```python
from build123d import *

# Parameters (mm, degrees)
BOSS_EXTRUDE1_DEPTH = 12.5
BOSS_EXTRUDE2_DEPTH = 7.5
BOSS_EXTRUDE3_DEPTH = 7.5
SKETCH5_W           = 44.45
SKETCH5_H           = 25
CUT_EXTRUDE1_DEPTH  = 10
CUT_EXTRUDE2_START  = -1.632728
SKETCH6_W           = 7.078863834
SKETCH6_H           = 10
CUT_EXTRUDE2_DEPTH  = 1.632728
BOSS_EXTRUDE4_DEPTH = 2
SKETCH8_R           = 1.5
CUT_EXTRUDE3_DEPTH  = 40


with BuildPart() as part:
    # Sketch1 → Boss-Extrude1 (new, symmetric)
    with BuildSketch(Plane.XY):
        with BuildLine():
            Line((-23.039431917, 7.577421516), (-13.039431917, 7.577421516))
            ThreePointArc((-13.039431917, 7.577421516), (0, -9.41875), (13.039431917, 7.577421516))
            Line((13.039431917, 7.577421516), (23.039431917, 7.577421516))
            Line((23.039431917, 7.577421516), (26.225, 2.38125))
            Line((26.225, 2.38125), (22.225, 2.38125))
            Line((22.225, 2.38125), (22.225, -17.61875))
            Line((22.225, -17.61875), (-22.225, -17.61875))
            Line((-22.225, -17.61875), (-22.225, 2.38125))
            Line((-22.225, 2.38125), (-26.225, 2.38125))
            Line((-26.225, 2.38125), (-23.039431917, 7.577421516))
        make_face()
    extrude(amount=BOSS_EXTRUDE1_DEPTH, both=True)

    # Sketch2 → Boss-Extrude2 (add)
    with BuildSketch(Plane.XY.offset(5)):
        with BuildLine():
            Line((-3.539431917, 5.944693506), (-3.539431917, 7.577421516))
            Line((-3.539431917, 7.577421516), (-13.039431917, 7.577421516))
            ThreePointArc((-13.039431917, 7.577421516), (0, -9.41875), (13.039431917, 7.577421516))
            Line((13.039431917, 7.577421516), (3.539431917, 7.577421516))
            Line((3.539431917, 7.577421516), (3.539431917, 5.944693506))
            ThreePointArc((3.539431917, 5.944693506), (0, 0.08125), (-3.539431917, 5.944693506))
        make_face()
    extrude(amount=BOSS_EXTRUDE2_DEPTH)

    # Sketch3 → Boss-Extrude3 (add)
    with BuildSketch(Plane.XY.offset(-5)):
        with BuildLine():
            Line((3.539431917, 7.577421516), (3.539431917, 5.944693506))
            ThreePointArc((3.539431917, 5.944693506), (0, 0.08125), (-3.539431917, 5.944693506))
            Line((-3.539431917, 5.944693506), (-3.539431917, 7.577421516))
            Line((-3.539431917, 7.577421516), (-13.039431917, 7.577421516))
            ThreePointArc((-13.039431917, 7.577421516), (0, -9.41875), (13.039431917, 7.577421516))
            Line((13.039431917, 7.577421516), (3.539431917, 7.577421516))
        make_face()
    extrude(amount=-BOSS_EXTRUDE3_DEPTH)

    # Sketch4 → Revolve1 (revolve)
    with BuildSketch(Plane(origin=(0, 4.08125, 0), x_dir=(1, 0, 0), z_dir=(0, 1, 0)), mode=Mode.PRIVATE) as revolve1_sk:
        Polygon((-4, -5), (-4, -3.5), (-6, -3.5), (-8.289431917, -5), align=None)
        Polygon((-4, 5), (-4, 3.5), (-6, 3.5), (-8.289431917, 5), align=None)
    revolve(revolve1_sk.sketch.rotate(Axis((0, 4.08125, 0), (0, 0, -1)), 27.765950742), axis=Axis((0, 4.08125, 0), (0, 0, -1)))

    # Sketch5 → Cut-Extrude1 (cut)
    with BuildSketch(Plane(origin=(0, 7.577421516, 0), x_dir=(1, 0, 0), z_dir=(0, 1, 0))):
        Rectangle(SKETCH5_W, SKETCH5_H)
    extrude(amount=CUT_EXTRUDE1_DEPTH, mode=Mode.SUBTRACT)

    # Sketch6 → Cut-Extrude2 (cut)
    with BuildSketch(Plane(origin=(0, 7.577421516, 0), x_dir=(1, 0, 0), z_dir=(0, 1, 0)).offset(CUT_EXTRUDE2_START)):
        Rectangle(SKETCH6_W, SKETCH6_H)
    extrude(amount=CUT_EXTRUDE2_DEPTH, mode=Mode.SUBTRACT)

    # Sketch7 → Boss-Extrude4 (add)
    with BuildSketch(Plane.XY.offset(12.5)):
        Polygon((-22.225, 2.38125), (-22.225, 7.577421516), (22.225, 7.577421516), (22.225, 2.38125), (22.225, -12.422578484), (-22.225, -12.422578484), align=None)
    boss_extrude4 = extrude(amount=-BOSS_EXTRUDE4_DEPTH)

    # Mirror1: Boss-Extrude4 across plane
    add(boss_extrude4.mirror(Plane.XY))

    # SurfaceCut1
    split(bisect_by=Plane(origin=(0, 0, -8.5), x_dir=(-1, 0, 0), z_dir=(0, 0, -1)), keep=Keep.BOTTOM)

    # Mirror2: part across plane


with BuildPart() as part_1:
    add(part.part)
    add(part.part.mirror(Plane(origin=(0, 0, -8.5), x_dir=(1, 0, 0), z_dir=(0, 0, -1))))

    # Sketch8 → Cut-Extrude3 (cut)
    with BuildSketch(Plane(origin=(0, 7.577421516, 0), x_dir=(1, 0, 0), z_dir=(0, 1, 0))):
        with Locations(Location((0, 0, 0), (0, 0, 180))):
            Circle(SKETCH8_R)
        with Locations(Location((0, 17, 0), (0, 0, 180))):
            Circle(SKETCH8_R)
    extrude(amount=-CUT_EXTRUDE3_DEPTH, mode=Mode.SUBTRACT)


solid = part_1.part
```
The listing builds one solid part. Answer for the finished solid, in the listing's coordinates (mm). A direction names the side the tool comes from. Coordinates: 2 decimals unless noted, no trailing zeros. Write each loop counter-clockwise with the first axis right and the second up, starting at its lowest first coordinate (ties: lowest second). Pieces come first, ordered by that corner, then holes. Notation, with made-up numbers: M 67.5,56 L 100.5,56 A34 ccw 100.5,91 Z; hole C -0.75,78 d4. An arc over 180 degrees is marked long. Use a Markdown table: item, result. Add a question column.
1. Straight lines are drawn through the part: line 1 along Z through (x, y) = (10, 4.5); line 2 along X through (y, z) = (2, -21.5) (3 decimals); line 3 along Z through (x, y) = (-1, -14). For each, find the intervals that lie inside material, in ascending order. Write a range as [from, to].
2. For a pull along Y with two mould halves and no side action, classify faces 1 (the flat face through (24.61, 5.016, -8.794)), 2 (the flat face through (3.539, 7, -24)), 3 (the cylindrical face through (-0.346, -9.414, -14.848)) as +Y half, -Y half, draft (parallel to the pull), parting line (faces both ways), or undercut.
3. Section A-A (x = 0) is taken. Count the separate pieces of the cut face and the enclosed holes in it, plus the area to 3 significant figures.
4. Section B-B (z = 0) is taken. Give the vertices of the cut face in (x, y) (3 decimals), plus the area to 3 significant figures.
5. Given P1, Ø1.8, axis at y = 7, z = -9, coming from the +X side; P2, Ø1.3, axis at y = 6.5, z = -24.5, coming from the -X side; P3, Ø12, axis at y = 1, z = 1.5, coming from the +X side (3 decimals), each flat-ended and moving along its own axis, determine where each tip first touches the part or whether it passes through.
6. Section C-C (y = -15.5) is taken. Give the vertices of the cut face in (x, z) (3 decimals), plus the area to 3 significant figures.
7. Section D-D (z = 6) is taken. Give the vertices of the cut face in (x, y) (3 decimals).
8. Which of the six approach directions +Z, -Z, +X, -X, +Y, -Y give full straight-line access (tool end or side, diameter ignored) to faces 4 (the flat face through (-24.655, 4.943, -8.794)), 5 (the flat face through (-1, 0, 3.5)), 6 (the cylindrical face through (-0.346, -9.414, 2.292))?
Data:
| question | item | result |
|---|---|---|
| 1 | line 1 | z = [-29.5, -22], [-12, -5], [5, 12.5] |
| 1 | line 2 | x = [-22.225, -13.339], [-7.233, -3.416], [3.416, 7.233], [13.339, 22.225] |
| 1 | line 3 | z = [-29.5, -18.12], [-15.88, -1.12], [1.12, 12.5] |
| 2 | face 1 | +Y half |
| 2 | face 2 | draft |
| 2 | face 3 | undercut |
| 3 | separate pieces | 3 |
| 3 | enclosed holes | 0 |
| 3 | area | 553 mm2 |
| 4 | outline | M -26.225,2.381 L -22.225,2.381 L -22.225,-17.619 L -1.5,-17.619 L -1.5,-9.335 A13.5 cw -13.039,7.577 L -23.039,7.577 Z; M 1.5,-17.619 L 22.225,-17.619 L 22.225,2.381 L 26.225,2.381 L 23.039,7.577 L 13.039,7.577 A13.5 cw 1.5,-9.335 Z |
| 4 | area | 741 mm2 |
| 5 | P1 | stops at x = 23.95 |
| 5 | P2 | stops at x = -24.1 |
| 5 | P3 | stops at x = 26.225 |
| 6 | outline | M -22.225,-29.5 L 22.225,-29.5 L 22.225,12.5 L -22.225,12.5 Z; hole C 0,-17 d3; hole C 0,0 d3 |
| 6 | area | 1,850 mm2 |
| 7 | outline | M -26.225,2.381 L -22.225,2.381 L -22.225,-17.619 L 22.225,-17.619 L 22.225,2.381 L 26.225,2.381 L 23.039,7.577 L 3.539,7.577 L 3.539,5.945 A4 cw long -3.539,5.945 L -3.539,7.577 L -23.039,7.577 Z |
| 8 | face 4 | +Z, -Z, -X, +Y |
| 8 | face 5 | +Y |
| 8 | face 6 | none |
